from build123d import *

# Parameters (mm, degrees)
SALIENTE_EXTRUIR1_DEPTH = 21.5
CORTAR_EXTRUIR1_DEPTH   = 0.01
CROQUIS3_R              = 1.5
SALIENTE_EXTRUIR2_DEPTH = 0.01
CROQUIS4_R              = 0.5
CORTAR_EXTRUIR2_DEPTH   = 0.5


with BuildPart() as part:
    # Croquis1 → Saliente-Extruir1 (new body)
    with BuildSketch(Plane.XY):
        with BuildLine():
            Line((0, 0), (-62, 0))
            ThreePointArc((-62, 0), (-63.497440295, 21), (-62, 42))
            Line((-62, 42), (0, 42))
            ThreePointArc((0, 42), (1.497440295, 21), (0, 0))
        make_face()
    extrude(amount=SALIENTE_EXTRUIR1_DEPTH)

    # Croquis2 → Cortar-Extruir1 (cut)
    with BuildSketch(Plane(origin=(0, 42, 0), x_dir=(1, 0, 0), z_dir=(0, 1, 0))):
        with BuildLine():
            Line((-47, -6.75), (-38.5, -6.75))
            ThreePointArc((-38.5, -6.75), (-34.5, -10.75), (-38.5, -14.75))
            Line((-38.5, -14.75), (-47, -14.75))
            ThreePointArc((-47, -14.75), (-51, -10.75), (-47, -6.75))
        make_face()
    extrude(amount=-CORTAR_EXTRUIR1_DEPTH, mode=Mode.SUBTRACT)

    # Croquis3 → Saliente-Extruir2 (add)
    with BuildSketch(Plane(origin=(0, 41.99, 0), x_dir=(1, 0, 0), z_dir=(0, 1, 0))):
        with Locations(Location((-38.5, -10.75, 0), (0, 0, 90))):
            Circle(CROQUIS3_R)
    extrude(amount=SALIENTE_EXTRUIR2_DEPTH)

    # Croquis4 → Cortar-Extruir2 (cut)
    with BuildSketch(Plane(origin=(0, 42, 0), x_dir=(1, 0, 0), z_dir=(0, 1, 0))):
        with Locations(Location((-56, -10.75, 0), (0, 0, 270))):
            Circle(CROQUIS4_R)
    extrude(amount=-CORTAR_EXTRUIR2_DEPTH, mode=Mode.SUBTRACT)

    # Croquis6 → Revolución1 (revolve)
    with BuildSketch(Plane(origin=(0, 21, 0), x_dir=(-1, 0, 0), z_dir=(0, -1, 0))):
        Polygon((25.502559705, -21.5), (25.502559705, -30), (24.502559705, -30), (23.592634119, -27.5), (22.592634119, -27.5), (13.802559705, -27.5), (13.802559705, -21.5), align=None)
    revolve(axis=Axis((-13.802559705, 21, 21.5), (0, 0, 1)))

    # Croquis9 → Revolución3 (revolve)
    with BuildSketch(Plane(origin=(0, 21, 0), x_dir=(1, 0, 0), z_dir=(0, 1, 0)), mode=Mode.PRIVATE) as revoluci_n3_sk:
        with BuildLine():
            Line((-13.802559705, -27.5), (-13.802559705, -30))
            ThreePointArc((-13.802559705, -30), (-18.810632516, -29.192650791), (-23.592634119, -27.5))
            Line((-23.592634119, -27.5), (-13.802559705, -27.5))
        make_face()
    revolve(revoluci_n3_sk.sketch.rotate(Axis((-13.802559705, 21, 27.5), (0, 0, 1)), 270), axis=Axis((-13.802559705, 21, 27.5), (0, 0, 1)))


solid = part.part
Verification items for the finished model (mm, model axes). A direction names the side the tool comes from. Coordinates: 2 decimals unless noted, no trailing zeros. Order: outer loops, then holes, each group sorted by start corner. A loop starts at its lowest first (then second) coordinate and runs counter-clockwise, first axis right, second up. Notation, with made-up numbers: M 75,18.5 L 112,18.5 A20 cw 112,40.5 Z; hole C 76.5,-33 d9. An arc over 180 degrees is marked long. One line per item, written item: value. Start each with the question number.
Item 1: Sectioned sample at B-B on z = 2.5. Record the cut outline in (x, y).
Item 2: Sectioned sample at C-C on y = 39.5. Record the cut outline in (x, z), then the cut area to 3 significant figures.
Item 3: Thickness scan on probe 1 along Z at (x, y) = (-56, 41.9); probe 2 along Z at (x, y) = (-45.5, 3); probe 3 along X at (y, z) = (41.8, 10.75). Record the ranges inside material, lowest first.
Item 4: Sectioned sample at D-D on z = 23. Record the cut outline in (x, y), then the cut area to 3 significant figures.
Item 5: Depth check by flat-ended pin: P1, Ø12, axis at x = -42.5, y = 5, coming from the +Z side; P2, Ø1.1, axis at x = -56, z = 11, coming from the +Y side. Enter the tip coordinate at first touch or a pass-through.
Item 6: Access from +Z, -Z, +X, -X, +Y, -Y to the whole of each face (thin tool, end or side, straight path). Record for faces 1 (the flat face through (-24.15, 24.41, 30)), 2 (the cylindrical face through (-12.28, 9.4, 25.81)).
Calculated:
1. outline: M -62,0 L 0,0 A148 ccw 0,42 L -62,42 A148 ccw Z
2. outline: M -62.34,0 L 0.34,0 L 0.34,21.5 L -62.34,21.5 Z
2. area: 1,350 mm^2
3. probe 1: 0 to 10.25, 11.25 to 21.5
3. probe 2: 0 to 21.5
3. probe 3: -62.03 to -56.5, -55.5 to 0.03
4. outline: C -13.8,21 d23.4
4. area: 430 mm^2
5. P1: z = 21.5
5. P2: y = 42
6. face 1: +Z, +X, -X, +Y, -Y
6. face 2: +Z
